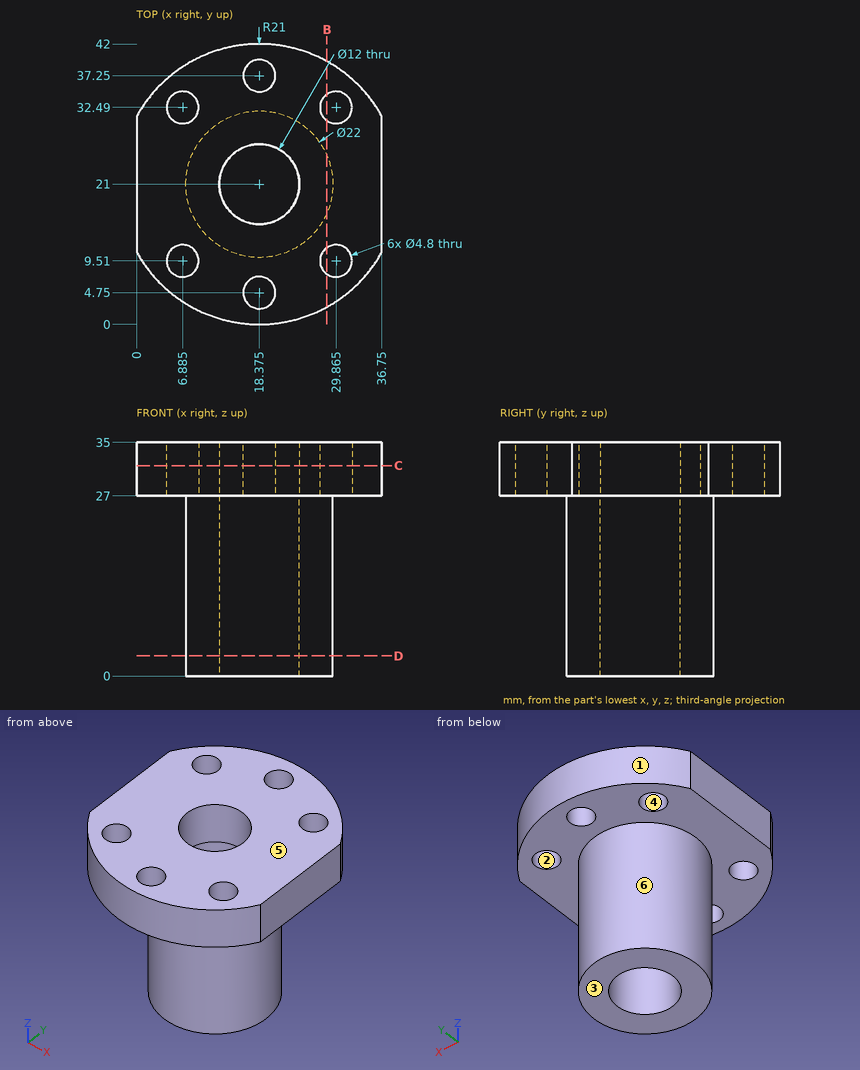
Source: three-view drawing plus pictorial views. Frame: mm from the lowest corner of the part. A direction names the side the tool comes from. Round coordinates to 2 decimals unless told otherwise and drop trailing zeros. Order: outer loops, then holes, each group sorted by start corner. A loop starts at its lowest first (then second) coordinate and runs counter-clockwise, first axis right, second up. Notation, with made-up numbers: (-37.5, -39) - (-11.5, -39) arc R30 ccw to (-11.5, 0) - close; hole circle Ø1 at (45, 58). An arc over 180 degrees is marked (long way). Answer in a Markdown table with one row per item.
Item 1: Section query B-B (x = 28.5). Return the cut outline in (y, z) (1 decimal).
Model answer:
| item | result |
|---|---|
| outline | (2.6, 27) - (7.5, 27) - (7.5, 35) - (2.6, 35) - close; (11.5, 27) - (16.7, 27) - (16.7, 0) - (25.3, 0) - (25.3, 27) - (30.5, 27) - (30.5, 35) - (11.5, 35) - close; (34.5, 27) - (39.4, 27) - (39.4, 35) - (34.5, 35) - close |
Item 2: Pin query (flat end, axial travel): pin 1 (10 mm diameter, centred on x = 26.5, y = 35, fed in from -Z); pin 2 (12 mm diameter, centred on x = 12.5, z = 9, fed in from -Y); pin 3 (4 mm diameter, centred on x = 27.5, z = 17, fed in from -Y). Return the tip coordinate at first contact, or that it passes through.
Model answer:
| item | result |
|---|---|
| pin 1 | stops at z = 27 |
| pin 2 | stops at y = 10 |
| pin 3 | stops at y = 12.62 |
Item 3: Reachability of the marked faces 5 and 6 from +Z, -Z, +X, -X, +Y, -Y: full face, straight path, thin tool, end or side. Return the list, or none.
Model answer:
| item | result |
|---|---|
| face 5 | +Z, +X, -X, +Y, -Y |
| face 6 | -Z |
Item 4: Section query C-C (z = 31.5). Give the number of separate pieces and of enclosed holes in the cut face, then the cut area to 3 significant figures.
Model answer:
| item | result |
|---|---|
| separate pieces | 1 |
| enclosed holes | 7 |
| area | 1,090 mm² |
Item 5: Section query D-D (z = 3). Return the cut outline in (x, y) (1 decimal), then the cut area to 3 significant figures.
Model answer:
| item | result |
|---|---|
| outline | circle Ø22 at (18.4, 21); hole circle Ø12 at (18.4, 21) |
| area | 267 mm² |
Item 6: Mould query, pull axis X, two halves, no side actions, for the marked faces 1, 2, 3 and 4. Classes: released by +X, released by -X, zero draft, split by the parting line, or undercut.
Model answer:
| item | result |
|---|---|
| face 1 | split by the parting line |
| face 2 | undercut |
| face 3 | zero draft |
| face 4 | undercut |
Item 7: Line query: line 1 (X direction, y = 33, z = 32); line 2 (Z direction, x = 9, y = 12.5); line 3 (Y direction, x = 18, z = 21.5). Output: solid intervals per line, ascending.
Model answer:
| item | result |
|---|---|
| line 1 | x = 1.14 to 4.54, 9.23 to 27.52, 32.21 to 35.61 |
| line 2 | z = 27 to 35 |
| line 3 | y = 10.01 to 15.01, 26.99 to 31.99 |
